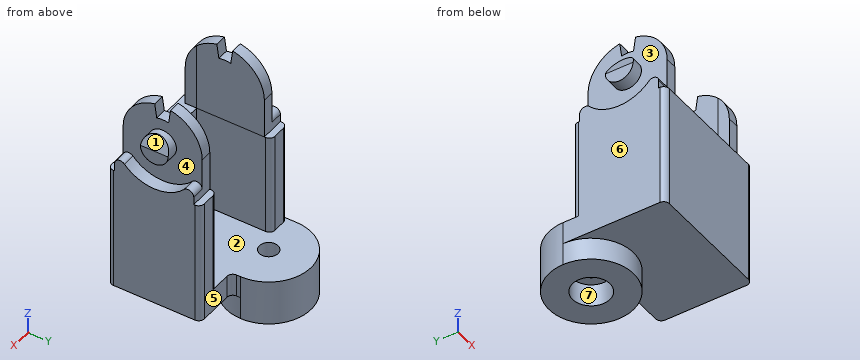
from build123d import *
from build123d.topology import SkipClean

# Parameters (mm, degrees)
SKETCH1_R           = 1.65
BOSS_EXTRUDE1_DEPTH = 40
CUT_EXTRUDE1_START  = -31.98
CUT_EXTRUDE1_DEPTH  = 31.98
SKETCH3_R           = 3.3
CUT_EXTRUDE2_DEPTH  = 4
CUT_EXTRUDE3_DEPTH  = 14
CUT_EXTRUDE4_REACH  = 51.576
SKETCH6_R           = 2.45
CUT_EXTRUDE5_DEPTH  = 2.25
CUT_EXTRUDE6_START  = -20.75
SKETCH6_2_R         = 2.45
CUT_EXTRUDE6_DEPTH  = 2.25
CUT_EXTRUDE7_START  = -9.45
CUT_EXTRUDE7_DEPTH  = 4.9


with BuildPart() as part:
    # Sketch1 → Boss-Extrude1 (new body)
    with BuildSketch(Plane.XY):
        with BuildLine():
            Line((8.48683607, -1.711916105), (14.51316393, -1.711916105))
            ThreePointArc((14.51316393, -1.711916105), (15.220270711, -2.004809324), (15.51316393, -2.711916105))
            Line((15.51316393, -2.711916105), (15.51316393, -17.131916105))
            ThreePointArc((15.51316393, -17.131916105), (15.220270711, -17.839022886), (14.51316393, -18.131916105))
            Line((14.51316393, -18.131916105), (-6.48683607, -18.131916105))
            ThreePointArc((-6.48683607, -18.131916105), (-7.193942851, -17.839022886), (-7.48683607, -17.131916105))
            Line((-7.48683607, -17.131916105), (-7.48683607, 0))
            ThreePointArc((-7.48683607, 0), (0, 7.48683607), (7.48683607, 0))
            Line((7.48683607, 0), (7.48683607, -0.711916105))
            ThreePointArc((7.48683607, -0.711916105), (7.779729289, -1.419022886), (8.48683607, -1.711916105))
        make_face()
        with Locations(Location((0, 0, 0), (0, 0, 180))):
            Circle(SKETCH1_R, mode=Mode.SUBTRACT)
    extrude(amount=BOSS_EXTRUDE1_DEPTH)

    # Sketch2 → Cut-Extrude1 (cut)
    with BuildSketch(Plane.XY.offset(40).offset(CUT_EXTRUDE1_START)):
        with BuildLine():
            Line((-3.22683607, -14.911916105), (-3.22683607, -2.711916105))
            ThreePointArc((-3.22683607, -2.711916105), (-3.519729289, -2.004809324), (-4.22683607, -1.711916105))
            Line((-4.22683607, -1.711916105), (-6.48683607, -1.711916105))
            ThreePointArc((-6.48683607, -1.711916105), (-7.193942851, -2.004809324), (-7.48683607, -2.711916105))
            Line((-7.48683607, -2.711916105), (-7.48683607, 0))
            ThreePointArc((-7.48683607, 0), (0, 7.48683607), (7.48683607, 0))
            Line((7.48683607, 0), (7.48683607, -0.711916105))
            ThreePointArc((7.48683607, -0.711916105), (7.779729289, -1.419022886), (8.48683607, -1.711916105))
            Line((8.48683607, -1.711916105), (12.25316393, -1.711916105))
            ThreePointArc((12.25316393, -1.711916105), (11.546057149, -2.004809324), (11.25316393, -2.711916105))
            Line((11.25316393, -2.711916105), (11.25316393, -14.911916105))
            Line((11.25316393, -14.911916105), (-3.22683607, -14.911916105))
        make_face()
    extrude(amount=CUT_EXTRUDE1_DEPTH, mode=Mode.SUBTRACT)

    # Sketch3 → Cut-Extrude2 (cut)
    with SkipClean():  # the faces are left unmerged after this step: merging them gives an invalid solid
        with BuildSketch(Plane(origin=(0, 0, 0), x_dir=(-1, 0, 0), z_dir=(0, 0, -1))):
            Circle(SKETCH3_R)
            with BuildLine():
                Line((-7.48683607, 0), (-7.48683607, -0.711916105))
                ThreePointArc((-7.48683607, -0.711916105), (-7.779729289, -1.419022886), (-8.48683607, -1.711916105))
                Line((-8.48683607, -1.711916105), (-14.51316393, -1.711916105))
                ThreePointArc((-14.51316393, -1.711916105), (-15.220270711, -2.004809324), (-15.51316393, -2.711916105))
                Line((-15.51316393, -2.711916105), (-15.51316393, -17.131916105))
                ThreePointArc((-15.51316393, -17.131916105), (-15.220270711, -17.839022886), (-14.51316393, -18.131916105))
                Line((-14.51316393, -18.131916105), (6.48683607, -18.131916105))
                ThreePointArc((6.48683607, -18.131916105), (7.193942851, -17.839022886), (7.48683607, -17.131916105))
                Line((7.48683607, -17.131916105), (7.48683607, 0))
                ThreePointArc((7.48683607, 0), (0, -7.48683607), (-7.48683607, 0))
            make_face()
        extrude(amount=-CUT_EXTRUDE2_DEPTH, mode=Mode.SUBTRACT)
    add(part.part.scale(1), mode=Mode.REPLACE)  # the faces are merged on a copy

    # Sketch4 → Cut-Extrude3 (cut)
    with BuildSketch(Plane.XY.offset(40)):
        Polygon((-3.22683607, -16.921916105), (-3.22683607, -2.921916105), (-7.48683607, -2.921916105), (-7.48683607, -1.711916105), (15.51316393, -1.711916105), (15.51316393, -2.921916105), (11.25316393, -2.921916105), (11.25316393, -16.921916105), (15.51316393, -16.921916105), (15.51316393, -18.131916105), (-7.48683607, -18.131916105), (-7.48683607, -16.921916105), align=None)
    extrude(amount=-CUT_EXTRUDE3_DEPTH, mode=Mode.SUBTRACT)

    # Cut-Extrude4: up to this face of the body (flat: up to its plane)
    cut_extrude4_end = Plane(part.part.faces().sort_by_distance((-7.48683607, -9.743748244, 21.544013895))[0])
    # Sketch5 → Cut-Extrude4 (cut, up to the picked face)
    with BuildSketch(Plane(origin=(15.51316393, 0, 0), x_dir=(0, 0, -1), z_dir=(1, 0, 0)), mode=Mode.PRIVATE) as cut_extrude4_sk1:
        with BuildLine():
            Line((-39.85857128, -8.521916105), (-37.324349662, -8.871916105))
            ThreePointArc((-37.324349662, -8.871916105), (-37.45, -9.921916105), (-37.324349662, -10.971916105))
            Line((-37.324349662, -10.971916105), (-39.85857128, -11.321916105))
            ThreePointArc((-39.85857128, -11.321916105), (-37.427188724, -15.34409279), (-33, -16.921916105))
            Line((-33, -16.921916105), (-40, -16.921916105))
            Line((-40, -16.921916105), (-40, -2.921916105))
            Line((-40, -2.921916105), (-33, -2.921916105))
            ThreePointArc((-33, -2.921916105), (-37.427188724, -4.49973942), (-39.85857128, -8.521916105))
        make_face()
    cut_extrude4_tool1 = split(extrude(cut_extrude4_sk1.sketch, amount=-CUT_EXTRUDE4_REACH, mode=Mode.PRIVATE), bisect_by=cut_extrude4_end, keep=Keep.BOTH, mode=Mode.PRIVATE)
    add(cut_extrude4_tool1.solids().sort_by(Axis((15.513164, -9.921916, 38.506526), (-1, 0, 0)))[0], mode=Mode.SUBTRACT)

    # Sketch6 → Cut-Extrude5 (cut)
    with BuildSketch(Plane(origin=(15.51316393, 0, 0), x_dir=(0, 0, -1), z_dir=(1, 0, 0))):
        with BuildLine():
            Line((-27.410724555, -2.921916105), (-31.314770045, -2.921916105))
            ThreePointArc((-31.314770045, -2.921916105), (-40.2, -9.921916105), (-31.314770045, -16.921916105))
            Line((-31.314770045, -16.921916105), (-27.410724555, -16.921916105))
            ThreePointArc((-27.410724555, -16.921916105), (-28.341237133, -16.288176042), (-28.092343512, -15.190208788))
            ThreePointArc((-28.092343512, -15.190208788), (-25.8, -9.921916105), (-28.092343512, -4.653623422))
            ThreePointArc((-28.092343512, -4.653623422), (-28.341237133, -3.555656168), (-27.410724555, -2.921916105))
        make_face()
        with Locations((-33, -9.921916105)):
            Circle(SKETCH6_R, mode=Mode.SUBTRACT)
    extrude(amount=-CUT_EXTRUDE5_DEPTH, mode=Mode.SUBTRACT)

    # Sketch6<2> → Cut-Extrude6 (cut)
    with BuildSketch(Plane(origin=(15.51316393, 0, 0), x_dir=(0, 0, -1), z_dir=(1, 0, 0)).offset(CUT_EXTRUDE6_START)):
        with BuildLine():
            Line((-27.410724555, -2.921916105), (-31.314770045, -2.921916105))
            ThreePointArc((-31.314770045, -2.921916105), (-40.2, -9.921916105), (-31.314770045, -16.921916105))
            Line((-31.314770045, -16.921916105), (-27.410724555, -16.921916105))
            ThreePointArc((-27.410724555, -16.921916105), (-28.341237133, -16.288176042), (-28.092343512, -15.190208788))
            ThreePointArc((-28.092343512, -15.190208788), (-25.8, -9.921916105), (-28.092343512, -4.653623422))
            ThreePointArc((-28.092343512, -4.653623422), (-28.341237133, -3.555656168), (-27.410724555, -2.921916105))
        make_face()
        with Locations((-33, -9.921916105)):
            Circle(SKETCH6_2_R, mode=Mode.SUBTRACT)
    extrude(amount=-CUT_EXTRUDE6_DEPTH, mode=Mode.SUBTRACT)

    # Sketch7 → Cut-Extrude7 (cut)
    with BuildSketch(Plane(origin=(0, -2.921916105, 0), x_dir=(1, 0, 0), z_dir=(0, 1, 0)).offset(CUT_EXTRUDE7_START)):
        Polygon((-7.48683607, -33), (-6.36183607, -35.45), (-7.48683607, -35.45), align=None)
        Polygon((15.51316393, -33), (15.51316393, -35.45), (14.38816393, -35.45), align=None)
    extrude(amount=CUT_EXTRUDE7_DEPTH, mode=Mode.SUBTRACT)


solid = part.part
The model under review builds one solid part; all positions refer to its coordinate system, in mm. Face numbers are marked on the shaded views. A direction names the side the tool comes from. Round coordinates to 2 decimals unless told otherwise and drop trailing zeros. Loops run counter-clockwise (first coordinate to the right, second up) from the corner with the lowest first, then second, coordinate; pieces in that order, holes last. Notation, with made-up numbers: (0, 36) -> (22, 36) arc R24 cw to (22, 67) -> close; hole circle Ø4 at (-5.5, 61.25). An arc over 180 degrees is marked (long way). Return JSON: item names as keys, results as strings.
(1) Add section B-B on z = 19. Write out the cut boundary in (x, y).
Solved:
{"outline": "(-7.49, -17.13) arc R1 ccw to (-6.49, -18.13) -> (14.51, -18.13) arc R1 ccw to (15.51, -17.13) -> (15.51, -2.71) arc R1 ccw to (14.51, -1.71) -> (12.25, -1.71) arc R1 ccw to (11.25, -2.71) -> (11.25, -14.91) -> (-3.23, -14.91) -> (-3.23, -2.71) arc R1 ccw to (-4.23, -1.71) -> (-6.49, -1.71) arc R1 ccw to (-7.49, -2.71) -> close"}
(2) Add section D-D on y = 6. Write out the cut boundary in (x, z), plus the area to 3 significant figures.
Solved:
{"outline": "(-4.48, 0) -> (4.48, 0) -> (4.48, 8.02) -> (-4.48, 8.02) -> close", "area": "71.8 mm2"}
(3) Add section C-C on y = -6.25. Write out the cut boundary in (x, z).
Solved:
{"outline": "(-7.49, 4) -> (-4.12, 4) -> (-4.12, 0) -> (4.12, 0) -> (4.12, 4) -> (15.51, 4) -> (15.51, 26.81) -> (13.26, 26.81) -> (13.26, 38.96) -> (11.25, 38.96) -> (11.25, 8.02) -> (-3.23, 8.02) -> (-3.23, 38.96) -> (-5.24, 38.96) -> (-5.24, 26.81) -> (-7.49, 26.81) -> close"}
(4) The part is to be moulded in two halves that separate along Y. For the marked faces 4, 5, 6 and 7, say which applies: released by +Y, released by -Y, zero draft, split by the parting line, or undercut.
Solved:
{"face 4": "undercut", "face 5": "released by +Y", "face 6": "zero draft", "face 7": "undercut"}
(5) For the marked faces 1, 2 and 3, list the 3-axis set-ups (+Z, -Z, +X, -X, +Y, -Y) from which the entire face can be reached by the end or side of a thin tool; tool diameter is ignored.
Solved:
{"face 1": "+Z, +X, +Y, -Y", "face 2": "+Z, +Y", "face 3": "-X"}
(6) For line 1 (X direction, y = -9, z = 9); line 2 (Y direction, x = 0, z = 6.85); line 3 (Y direction, x = 0, z = 3.1), list the stretches that pass through material, from the lowest coordinate up.
Solved:
{"line 1": "-7.49 to -3.23, 11.25 to 15.51", "line 2": "-18.13 to -1.65, 1.65 to 7.49", "line 3": "-7.49 to -3.3, 3.3 to 7.49"}
(7) Add section A-A on x = 0. Write out the cut boundary in (y, z), plus the area to 3 significant figures.
Solved:
{"outline": "(-18.13, 4) -> (-7.49, 4) -> (-7.49, 0) -> (-3.3, 0) -> (-3.3, 4) -> (-1.65, 4) -> (-1.65, 8.02) -> (-14.91, 8.02) -> (-14.91, 26) -> (-18.13, 26) -> close; (1.65, 4) -> (3.3, 4) -> (3.3, 0) -> (7.49, 0) -> (7.49, 8.02) -> (1.65, 8.02) -> close", "area": "181 mm2"}
(8) For pin 1 (3.5 mm diameter, centred on x = 13, z = 28.5, fed in from -Y); pin 2 (0.6 mm diameter, centred on y = -16.5, z = 30.5, fed in from +X); pin 3 (4 mm diameter, centred on x = 0, y = 0, fed in from -Z); pin 4 (5 mm diameter, centred on x = 2.5, z = 29.5, fed in from -Y), all flat-tipped, find the tip position at first contact; note any pin that passes through.
Solved:
{"pin 1": "y = -16.92", "pin 2": "x = 13.26", "pin 3": "z = 4", "pin 4": "through"}
